from build123d import *

# Parameters (mm, degrees)
BOX036_W     = 9
BOX036_H     = 1.5
BOX036_DEPTH = 2
BOX037_W     = 9
BOX037_H     = 1.5
BOX037_DEPTH = 2
BOX006_W     = 39
BOX006_H     = 8
BOX006_DEPTH = 2
BOX005_W     = 38
BOX005_H     = 10
BOX005_DEPTH = 3


with BuildPart() as cubo036:
    # Box036 → Box036 (new body)
    with BuildSketch(Plane(origin=(-36, 63.25, 45), x_dir=(1, 0, 0), z_dir=(0, 0, 1))):
        with Locations((4.5, 0.75)):
            Rectangle(BOX036_W, BOX036_H)
    extrude(amount=BOX036_DEPTH)


with BuildPart() as cubo037:
    # Box037 → Box037 (new body)
    with BuildSketch(Plane(origin=(-36, 55.25, 45), x_dir=(1, 0, 0), z_dir=(0, 0, 1))):
        with Locations((4.5, 0.75)):
            Rectangle(BOX037_W, BOX037_H)
    extrude(amount=BOX037_DEPTH)


with BuildPart() as cubo006:
    # Box006 → Box006 (new body)
    with BuildSketch(Plane(origin=(-37, 56, 45), x_dir=(1, 0, 0), z_dir=(0, 0, 1))):
        with Locations((19.5, 4)):
            Rectangle(BOX006_W, BOX006_H)
    extrude(amount=BOX006_DEPTH)


with BuildPart() as fusion002019:
    # Box005 → Box005 (new body)
    with BuildSketch(Plane(origin=(-37, 55, 45), x_dir=(1, 0, 0), z_dir=(0, 0, 1))):
        with Locations((19, 5)):
            Rectangle(BOX005_W, BOX005_H)
    extrude(amount=BOX005_DEPTH)

    # Cut054: cut Cubo006
    add(cubo006.part, mode=Mode.SUBTRACT)


with BuildPart() as fusion002019_1:
    # Cut054 placement: moved
    add(fusion002019.part.moved(Location((1, 0, 0))))

    # Fusion002019: union Cubo036, Cubo037
    add(cubo036.part)
    add(cubo037.part)


solid = fusion002019_1.part
Geometry check sheet. Reference: the model listing, model coordinates, mm. A direction names the side the tool comes from. Give positions to 0.01 mm unless a question says otherwise; leave off trailing zeros. Order: outer loops, then holes, each group sorted by start corner. A loop starts at its lowest first (then second) coordinate and runs counter-clockwise, first axis right, second up.
1. Sectioned sample at A-A (z = 46.25). Record the boundary of the cut face in (x, y), then the cut area to 3 significant figures.
Completed:
outline: (-36, 55) - (2, 55) - (2, 56) - (-27, 56) - (-27, 56.75) - (-36, 56.75) - close; (-36, 63.25) - (-27, 63.25) - (-27, 64) - (2, 64) - (2, 65) - (-36, 65) - close
area: 89.5 mm2
2. Depth check by flat-ended pin: pin 1 (0.8 mm diameter, centred on y = 56.5, z = 45.5, fed in from +X). Enter the tip coordinate at first touch or a pass-through.
Completed:
pin 1: stops at x = -27
3. Draft check along Y on faces 4 (the face through (-36, 59.9, 47.5)), 5 (the face through (-13, 64, 46)), 6 (the face through (-17, 65, 46)). Enter one of: pulls with the +Y half, pulls with the -Y half, needs draft (parallel to the pull), parting line crosses it, or undercut.
Completed:
face 4: needs draft
face 5: undercut
face 6: pulls with the +Y half
4. Scan lines: line 1 (Y direction, x = 0, z = 45.3); line 2 (Y direction, x = -29.5, z = 45.9); line 3 (Z direction, x = -20.5, y = 59.5). Record each from-to range of solid material in increasing order.
Completed:
line 1: y = 55 to 56, 64 to 65
line 2: y = 55 to 56.75, 63.25 to 65
line 3: z = 47 to 48
5. Sectioned sample at B-B (x = -4). Record the boundary of the cut face in (y, z), then the cut area to 3 significant figures.
Completed:
outline: (55, 45) - (56, 45) - (56, 47) - (64, 47) - (64, 45) - (65, 45) - (65, 48) - (55, 48) - close
area: 14.0 mm2
6. Sectioned sample at C-C (y = 61.25). Record the boundary of the cut face in (x, z).
Completed:
outline: (-36, 47) - (2, 47) - (2, 48) - (-36, 48) - close
7. Access from +Z, -Z, +X, -X, +Y, -Y to the whole of each face (thin tool, end or side, straight path). Record for faces 1 (the face through (-21.5, 64.3, 45)), 2 (the face through (-13, 56, 46)), 3 (the face through (-32, 63.25, 46)).
Completed:
face 1: -Z, +X, -X, +Y, -Y
face 2: -Z, +X
face 3: -Z, +X, -X
